```python
from build123d import *

# Parameters (mm, degrees)
SKETCH_W        = 40
SKETCH_H        = 24
PAD_DEPTH       = 3
SKETCH001_W     = 6
SKETCH001_H     = 24
PAD001_DEPTH    = 25
POCKET_DEPTH    = 6
POCKET001_DEPTH = 6
SKETCH005_R     = 1.5
POCKET002_DEPTH = 24.001
FILLET_R        = 3


with BuildPart() as part:
    # Sketch → Pad (new body)
    with BuildSketch(Plane.XY):
        Rectangle(SKETCH_W, SKETCH_H)
    extrude(amount=PAD_DEPTH)

    # Sketch001 (on Face6 of Pad) → Pad001 (join)
    with BuildSketch(Plane.XY.offset(3)):
        with Locations((-17, 0)):
            Rectangle(SKETCH001_W, SKETCH001_H)
        with Locations((17, 0)):
            Rectangle(SKETCH001_W, SKETCH001_H)
    extrude(amount=PAD001_DEPTH)

    # Sketch002 (on Face9 of Pad001) → Pocket (cut)
    with BuildSketch(Plane.YZ.offset(20)):
        with BuildLine():
            Line((-3.5, 28), (3.5, 28))
            Line((3.5, 28), (3.5, 13.999995))
            ThreePointArc((-3.5, 13.999984), (5e-06, 10.5), (3.5, 13.999995))
            Line((-3.5, 13.999984), (-3.5, 28))
        make_face()
    extrude(amount=-POCKET_DEPTH, mode=Mode.SUBTRACT)

    # Sketch004 (on Face12 of Pocket) → Pocket001 (cut)
    with BuildSketch(Plane(origin=(-20, 0, 0), x_dir=(0, -1, 0), z_dir=(-1, 0, 0))):
        with BuildLine():
            Line((-7.65, 28), (7.65, 28))
            Line((7.65, 28), (7.65, 14))
            ThreePointArc((-7.65, 14), (0, 6.35), (7.65, 14))
            Line((-7.65, 14), (-7.65, 28))
        make_face()
    extrude(amount=-POCKET001_DEPTH, mode=Mode.SUBTRACT)

    # Sketch005 (on Face10 of Pocket001) → Pocket002 (cut, through all)
    with BuildSketch(Plane.XZ.offset(12)):
        with Locations((17, 21)):
            Circle(SKETCH005_R)
        with Locations((-17, 24)):
            Circle(SKETCH005_R)
    extrude(amount=-POCKET002_DEPTH, mode=Mode.SUBTRACT)

    # Fillet
    fillet_edges = [part.edges().sort_by_distance(p)[0] for p in [
        (-14, 0, 3),
        (14, 0, 3),
    ]]
    fillet(fillet_edges, radius=FILLET_R)


solid = part.part
```
Geometry: final body of the model. Coordinates: model frame, mm. A direction names the side the tool comes from. Coordinates: 2 decimals unless noted, no trailing zeros. Write each loop counter-clockwise with the first axis right and the second up, starting at its lowest first coordinate (ties: lowest second). Pieces come first, ordered by that corner, then holes. Notation, with made-up numbers: M 78,-9.5 L 85,-9.5 A14 ccw 85,-0.5 Z; hole C -18.5,-38 d1. An arc over 180 degrees is marked long. Answer as CSV lines item,"result". Start each with the question number.
Q1. Line query: line 1 (Z direction, x = -17, y = 11.15); line 2 (Z direction, x = 17, y = -6.25); line 3 (Y direction, x = 15.5, z = 17). Output: solid intervals per line, ascending. Write a range as from..to.
Q2. Cut plane C-C on z = 21. Return the cut outline in (x, y).
Q3. Cut plane D-D on y = -8.75. Return the cut outline in (x, z), then the cut area to 3 significant figures.
Q4. Reachability of faces 1 (the flat face through (-14, -8, 17)), 2 (the flat face through (0, 0, 0)), 3 (the cylindrical face through (-17.04, 0.17, 6.35)) from +Z, -Z, +X, -X, +Y, -Y: full face, straight path, thin tool, end or side. Return the list, or none.
Q5. Cut plane B-B on z = 26.25. Return the cut outline in (x, y), then the cut area to 3 significant figures.
Q6. Cut plane A-A on x = -17. Return the cut outline in (y, z), then the cut area to 3 significant figures.
Q7. Mould query, pull axis Y, two halves, no side actions, for faces 4 (the flat face through (17, 3.5, 23)), 5 (the flat face through (14, 5, 17)), 6 (the flat face through (0, 12, 1)). Classes: released by +Y, released by -Y, zero draft, split by the parting line, or undercut.
Q8. Pin query (flat end, axial travel): P1, Ø10, axis at x = 6, z = 6.5, coming from the -Y side; P2, Ø1.8, axis at x = -17, z = 24, coming from the +Y side; P3, Ø5, axis at x = 13.5, y = -0.5, coming from the +Z side; P4, Ø5, axis at y = -1.5, z = 10, coming from the -X side. Return the tip coordinate at first contact, or that it passes through.
Findings below:
1,line 1,"z = 0..22.5, 25.5..28"
1,line 2,"z = 0..19.5, 22.5..28"
1,line 3,"y = -12..-3.5, 3.5..12"
2,outline,"M -20,-12 L -14,-12 L -14,-7.65 L -20,-7.65 Z; M -20,7.65 L -14,7.65 L -14,12 L -20,12 Z; M 14,-12 L 15.5,-12 L 15.5,-3.5 L 14,-3.5 Z; M 14,3.5 L 15.5,3.5 L 15.5,12 L 14,12 Z; M 18.5,-12 L 20,-12 L 20,-3.5 L 18.5,-3.5 Z; M 18.5,3.5 L 20,3.5 L 20,12 L 18.5,12 Z"
3,outline,"M -20,0 L 20,0 L 20,28 L 14,28 L 14,6 A3 cw 11,3 L -11,3 A3 cw -14,6 L -14,28 L -20,28 Z; hole C -17,24 d3; hole C 17,21 d3"
3,area,"410 mm2"
4,face 1,"+Z, +Y, -Y"
4,face 2,"-Z, +X, -X, +Y, -Y"
4,face 3,"+Z, -X"
5,outline,"M -20,-12 L -14,-12 L -14,-7.65 L -20,-7.65 Z; M -20,7.65 L -14,7.65 L -14,12 L -20,12 Z; M 14,-12 L 20,-12 L 20,-3.5 L 14,-3.5 Z; M 14,3.5 L 20,3.5 L 20,12 L 14,12 Z"
5,area,"154 mm2"
6,outline,"M -12,0 L 12,0 L 12,22.5 L 7.65,22.5 L 7.65,14 A7.65 cw -7.65,14 L -7.65,22.5 L -12,22.5 Z; M -12,25.5 L -7.65,25.5 L -7.65,28 L -12,28 Z; M 7.65,25.5 L 12,25.5 L 12,28 L 7.65,28 Z"
6,area,"340 mm2"
7,face 4,"undercut"
7,face 5,"zero draft"
7,face 6,"released by +Y"
8,P1,"stops at y = -12"
8,P2,"passes through"
8,P3,"stops at z = 12.12"
8,P4,"stops at x = 14"
